```python
from build123d import *

# Parameters (mm, degrees)
SKETCH1_W           = 16
SKETCH1_H           = 16
SKETCH1_W_2         = 12
SKETCH1_H_2         = 12
BOSS_EXTRUDE1_DEPTH = 250
FILLET1_R           = 1
SKETCH2_R           = 2.5
CUT_EXTRUDE1_DEPTH  = 16
SKETCH3_R           = 2.5
CUT_EXTRUDE2_DEPTH  = 16
SKETCH4_R           = 2.5
CUT_EXTRUDE3_DEPTH  = 16
SKETCH5_R           = 2.5
CUT_EXTRUDE4_DEPTH  = 16


with BuildPart() as part:
    # Sketch1 → Boss-Extrude1 (new body)
    with BuildSketch(Plane(origin=(0, 0, 0), x_dir=(1, 0, 0), z_dir=(0, 1, 0))):
        with Locations((-0.059056614, 0.224719101)):
            Rectangle(SKETCH1_W, SKETCH1_H)
        with Locations((-0.059056614, 0.224719101)):
            Rectangle(SKETCH1_W_2, SKETCH1_H_2, mode=Mode.SUBTRACT)
    extrude(amount=BOSS_EXTRUDE1_DEPTH)

    # Fillet1
    fillet1_edges = [part.edges().sort_by_distance(p)[0] for p in [
        (-8.059056614, 125, -8.224719101),
        (7.940943386, 125, -8.224719101),
        (7.940943386, 125, 7.775280899),
        (-8.059056614, 125, 7.775280899),
    ]]
    fillet(fillet1_edges, radius=FILLET1_R)

    # Sketch2 → Cut-Extrude1 (cut)
    with BuildSketch(Plane.XY.offset(7.775280899)):
        with Locations((-0.059056614, 8)):
            Circle(SKETCH2_R)
    extrude(amount=-CUT_EXTRUDE1_DEPTH, mode=Mode.SUBTRACT)

    # Sketch3 → Cut-Extrude2 (cut)
    with BuildSketch(Plane.XY.offset(7.775280899)):
        with Locations((-0.059056614, 242)):
            Circle(SKETCH3_R)
    extrude(amount=-CUT_EXTRUDE2_DEPTH, mode=Mode.SUBTRACT)

    # Sketch4 → Cut-Extrude3 (cut)
    with BuildSketch(Plane.ZY.offset(8.059056614)):
        with Locations((-0.224719101, 24)):
            Circle(SKETCH4_R)
        with Locations((-0.224719101, 226)):
            Circle(SKETCH4_R)
    extrude(amount=-CUT_EXTRUDE3_DEPTH, mode=Mode.SUBTRACT)

    # Sketch5 → Cut-Extrude4 (cut)
    with BuildSketch(Plane.XY.offset(7.775280899)):
        with Locations((-0.059056614, 125)):
            Circle(SKETCH5_R)
    extrude(amount=-CUT_EXTRUDE4_DEPTH, mode=Mode.SUBTRACT)


solid = part.part
```
Geometry check sheet. Reference: the model listing, model coordinates, mm. A direction names the side the tool comes from. Give positions to 0.01 mm unless a question says otherwise; leave off trailing zeros. Order: outer loops, then holes, each group sorted by start corner. A loop starts at its lowest first (then second) coordinate and runs counter-clockwise, first axis right, second up. Notation, with made-up numbers: (-20.75, -17) -> (-2.75, -17) arc R7 cw to (-2.75, -7) -> close; hole circle Ø11 at (-26.5, 69). An arc over 180 degrees is marked (long way). Write each question's results on one line, items separated by ' | '. Start each with the question number.
(1) Sectioned sample at A-A (y = 242). Enter the section's corners in (x, z).
(2) Access from +Z, -Z, +X, -X, +Y, -Y to the whole of each face (thin tool, end or side, straight path). Record for faces 1 (the face through (-8.059, 123, 0)), 2 (the face through (5.941, 123, 0)).
(3) Mould release check, pull along Y, two halves, no side actions. Record for faces 3 (the face through (-3, 123, -6.225)), 4 (the face through (7, 250, 0)), 5 (the face through (-0.38, 127.48, -7.21)): pulls with the +Y half, pulls with the -Y half, needs draft (parallel to the pull), parting line crosses it, or undercut.
(4) Scan lines: line 1 (Z direction, x = 4.25, y = 96); line 2 (X direction, y = 147.5, z = 1); line 3 (Z direction, x = 7, y = 20.5). Record each from-to range of solid material in increasing order.
(5) Sectioned sample at B-B (y = 202.5). Enter the section's corners in (x, z).
Answer below:
1) outline: (-8.06, -7.22) arc R1 ccw to (-7.06, -8.22) -> (-2.56, -8.22) -> (-2.56, -6.22) -> (-6.06, -6.22) -> (-6.06, 5.78) -> (-2.56, 5.78) -> (-2.56, 7.78) -> (-7.06, 7.78) arc R1 ccw to (-8.06, 6.78) -> close; (2.44, -8.22) -> (6.94, -8.22) arc R1 ccw to (7.94, -7.22) -> (7.94, 6.78) arc R1 ccw to (6.94, 7.78) -> (2.44, 7.78) -> (2.44, 5.78) -> (5.94, 5.78) -> (5.94, -6.22) -> (2.44, -6.22) -> close
2) face 1: +Z, -Z, -X, +Y, -Y | face 2: +Y, -Y
3) face 3: needs draft | face 4: pulls with the +Y half | face 5: undercut
4) line 1: -8.22 to -6.22, 5.78 to 7.78 | line 2: -8.06 to -6.06, 5.94 to 7.94 | line 3: -8.22 to 7.77
5) outline: (-8.06, -7.22) arc R1 ccw to (-7.06, -8.22) -> (6.94, -8.22) arc R1 ccw to (7.94, -7.22) -> (7.94, 6.78) arc R1 ccw to (6.94, 7.78) -> (-7.06, 7.78) arc R1 ccw to (-8.06, 6.78) -> close; hole (-6.06, -6.22) -> (5.94, -6.22) -> (5.94, 5.78) -> (-6.06, 5.78) -> close
